Autodesk Inventor part; units mm, degrees
ref_plane "C3_XY" through (130, 0, 0) normal (-1, 0, 0) x (0, 0, -1)
ref_plane "C3_YZ" through (130, 0, 0) normal (0, 0, -1) x (0, -1, 0)
ref_plane "C3_ZX" through (130, 0, 0) normal (0, -1, 0) x (-1, 0, 0)
sketch "Sketch_1" plane through (0, 0, 0) normal (0, 0, 1) x (1, 0, 0)
  line L0 (130, 0) -> (0, 0)
  line L1 (0, 0) -> (0, 3.5)
  line L2 (0, 3.5) -> (0.6062, 4.55)
  line L3 (0.6062, 4.55) -> (129.3938, 4.55)
  line L4 (129.3938, 4.55) -> (130, 3.5)
  line L5 (130, 3.5) -> (130, 0)
  line L6 (130, 0) -> (0, 0)
revolve "Revolution1" add sketch "Sketch_1" angle 360 about axis through (130, 0, 0) along (1, 0, 0)
sketch "Sketch_2" plane through (0, 0, 0) normal (1, 0, 0) x (0, 1, 0)
  line L0 (7, 7) -> (-7, 7)
  line L1 (-7, 7) -> (-7, -7)
  line L2 (-7, -7) -> (7, -7)
  line L3 (7, -7) -> (7, 7)
  line L4 (-2.0207, 3.5) -> (-4.0415, 0)
  line L5 (-4.0415, 0) -> (-2.0207, -3.5)
  line L6 (-2.0207, -3.5) -> (2.0207, -3.5)
  line L7 (2.0207, -3.5) -> (4.0415, 0)
  line L8 (4.0415, 0) -> (2.0207, 3.5)
  line L9 (2.0207, 3.5) -> (-2.0207, 3.5)
extrude "Extrusion1" cut sketch "Sketch_2" along normal blind 130
sketch "Sketch3" plane through (0, 0, 0) normal (-1, 0, 0) x (0, 0, 1)
  point P0 (0, 0)
hole "Hole1" at (0, 0, 0) direction (1, 0, 0) diameter 2.459 depth 8.2901 tip angle 120 countersink diameter 3 countersink angle 90
sketch "Sketch4" plane through (130, 0, 0) normal (1, 0, 0) x (0, 0, -1)
  point P0 (0, 0)
hole "Hole2" at (130, 0, 0) direction (-1, 0, 0) diameter 2.459 depth 8.2901 tip angle 120 countersink diameter 3 countersink angle 90
ref_plane "C3_XY" through (130, 0, 0) normal (-1, 0, 0) x (0, 0, -1)
ref_plane "C3_YZ" through (130, 0, 0) normal (0, 0, -1) x (0, -1, 0)
ref_plane "C3_ZX" through (130, 0, 0) normal (0, -1, 0) x (-1, 0, 0)
properties part number "SLSBF7-130-M3-N3"
The model under review builds one solid part; all positions refer to its coordinate system, in mm. A direction names the side the tool comes from. Round coordinates to 2 decimals unless told otherwise and drop trailing zeros. Write each loop counter-clockwise with the first axis right and the second up, starting at its lowest first coordinate (ties: lowest second). Pieces come first, ordered by that corner, then holes. Notation, with made-up numbers: M 33,44 L 48,44 A9 cw 48,58 Z; hole C -33,-13 d8. An arc over 180 degrees is marked long. Use CSV: the item, a comma, the result in double quotes. Start each with the question number.
(1) For line 1 along Z through (x, y) = (126, 0); line 2 along Y through (x, z) = (4.25, 0); line 3 along X through (y, z) = (3.75, 0), list the stretches that pass through material, from the lowest coordinate up.
(2) Tool access review of faces 1 (the face through (125.664, 0.748, 0.976)), 2 (the face through (4.336, 0.748, -0.976)), 3 (the face through (130, 0, -2)): name each direction out of +Z, -Z, +X, -X, +Y, -Y from which nothing blocks a thin tool from reaching the whole face with its end or side.
(3) Clearance check with flat-ended pins moving along their axes: P1, Ø1.5, axis at y = 0, z = 0, coming from the +X side; P2, Ø2, axis at y = 0, z = 0, coming from the -X side. State where each tip first meets the part, or that it passes through.
(4) The part is to be moulded in two halves that separate along Z. For faces 4 (the face through (64.09, 3.045, 1.726)), 5 (the face through (64.09, -3.045, -1.726)), 6 (the face through (121, 0, 0)), say which applies: +Z half, -Z half, draft (parallel to the pull), parting line (faces both ways), or undercut.
(5) We need section A-A, the plane x = 32.5. State the section outline as (y, z) points.
Findings:
1,line 1,"-3.5 to -1.23, 1.23 to 3.5"
1,line 2,"-4.04 to -1.23, 1.23 to 4.04"
1,line 3,"0.14 to 129.86"
2,face 1,"+X"
2,face 2,"-X"
2,face 3,"+Z, -Z, +X, +Y, -Y"
3,P1,"x = 121.43"
3,P2,"x = 8.42"
4,face 4,"+Z half"
4,face 5,"-Z half"
4,face 6,"undercut"
5,outline,"M -4.04,0 L -2.02,-3.5 L 2.02,-3.5 L 4.04,0 L 2.02,3.5 L -2.02,3.5 Z"
